Design review of the part built by this model. Coordinates are the model's own, in mm. Coordinates: 2 decimals unless noted, no trailing zeros. Order: outer loops, then holes, each group sorted by start corner. A loop starts at its lowest first (then second) coordinate and runs counter-clockwise, first axis right, second up.
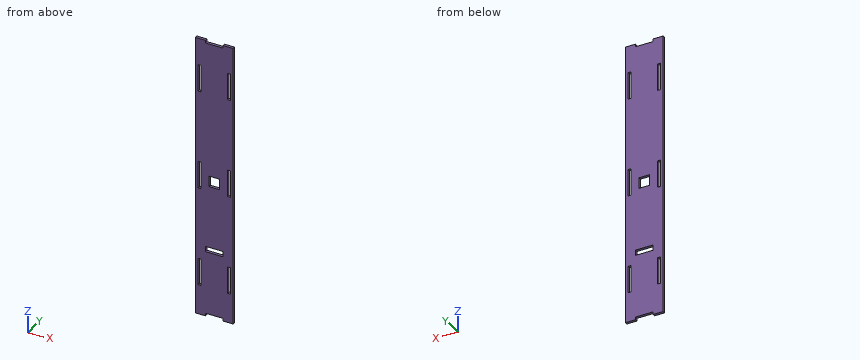
from build123d import *

# Parameters (mm, degrees)
SKETCH1_W           = 3
SKETCH1_H           = 30
SKETCH1_W_2         = 12
SKETCH1_H_2         = 12
SKETCH1_W_3         = 20
SKETCH1_H_3         = 6
BOSS_EXTRUDE1_DEPTH = 3


with BuildPart() as part:
    # Sketch1 → Boss-Extrude1 (new body)
    with BuildSketch(Plane(origin=(0, 0, 0), x_dir=(1, 0, 0), z_dir=(0, 1, 0))):
        Polygon((0, 313), (0, 0), (11, 0), (11, 3), (31, 3), (31, 0), (42, 0), (42, 313), (31, 313), (31, 310), (11, 310), (11, 313), align=None)
        with Locations((4.5, 45)):
            Rectangle(SKETCH1_W, SKETCH1_H, mode=Mode.SUBTRACT)
        with Locations((4.5, 155)):
            Rectangle(SKETCH1_W, SKETCH1_H, mode=Mode.SUBTRACT)
        with Locations((37.5, 45)):
            Rectangle(SKETCH1_W, SKETCH1_H, mode=Mode.SUBTRACT)
        with Locations((37.5, 155)):
            Rectangle(SKETCH1_W, SKETCH1_H, mode=Mode.SUBTRACT)
        with Locations((21, 159)):
            Rectangle(SKETCH1_W_2, SKETCH1_H_2, mode=Mode.SUBTRACT)
        with Locations((4.5, 265)):
            Rectangle(SKETCH1_W, SKETCH1_H, mode=Mode.SUBTRACT)
        with Locations((21, 237)):
            Rectangle(SKETCH1_W_3, SKETCH1_H_3, mode=Mode.SUBTRACT)
        with Locations((37.5, 265)):
            Rectangle(SKETCH1_W, SKETCH1_H, mode=Mode.SUBTRACT)
    extrude(amount=BOSS_EXTRUDE1_DEPTH)


solid = part.part
1. Add section B-B (z = -274.5). Give the boundary of the cut face in (x, y), and give its area (3 significant figures).
2. Add section C-C (y = 1.6). State how many separate pieces and enclosed holes the cut face has, and give its area (3 significant figures).
3. To check wall thickness, follow line 1 (Z direction, x = 15.5, y = 0.65); line 2 (Z direction, x = 36.5, y = 0.6); line 3 (X direction, y = 1.7, z = -266). State the ranges of each line that lie inside material, in increasing order.
4. Insertion check: pin 1 (0.9 mm diameter, centred on x = 24, y = 2, fed in from +Z). The pin has a flat end and moves straight along its axis. Give the tip position at first contact, or say it passes through.
5. Add section A-A (x = 22.5). Give the boundary of the cut face in (y, z).
Solution:
1. outline: (0, 0) - (3, 0) - (3, 3) - (0, 3) - close; (6, 0) - (36, 0) - (36, 3) - (6, 3) - close; (39, 0) - (42, 0) - (42, 3) - (39, 3) - close
1. area: 108 mm2
2. separate pieces: 1
2. enclosed holes: 8
2. area: 12,200 mm2
3. line 1: z = -310 to -240, -234 to -165, -153 to -3
3. line 2: z = -313 to -280, -250 to -170, -140 to -60, -30 to 0
3. line 3: x = 0 to 3, 6 to 36, 39 to 42
4. pin 1: stops at z = -3
5. outline: (0, -310) - (3, -310) - (3, -240) - (0, -240) - close; (0, -234) - (3, -234) - (3, -165) - (0, -165) - close; (0, -153) - (3, -153) - (3, -3) - (0, -3) - close
